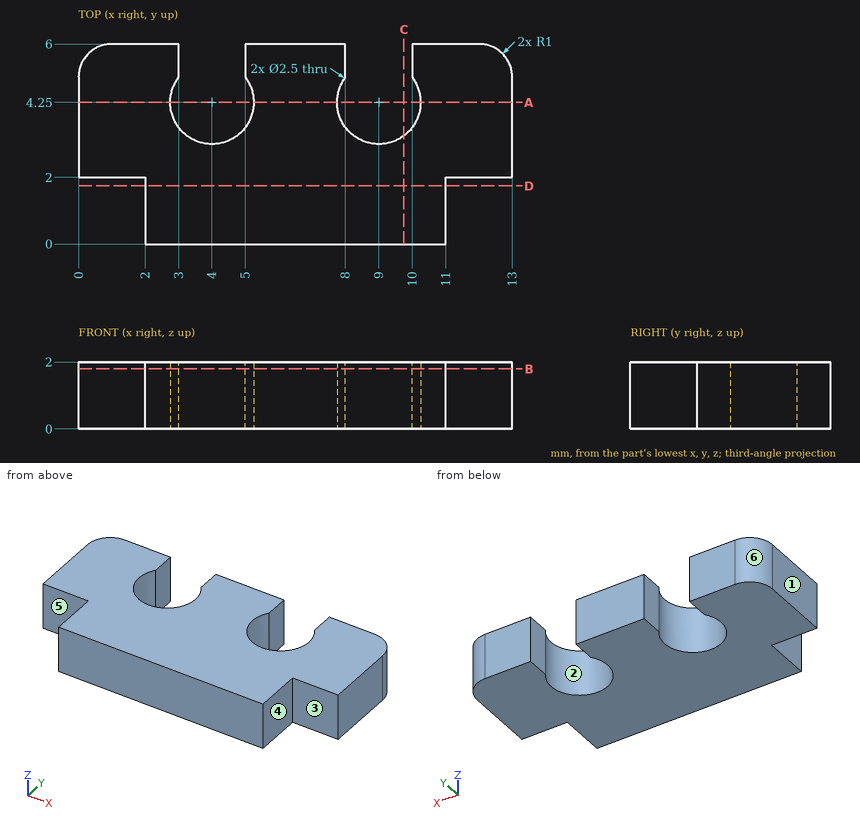
Geometry: see drawing. Coordinates: mm, zero at the bounding-box minimum. A direction names the side the tool comes from. Coordinates: 2 decimals unless noted, no trailing zeros. Order: outer loops, then holes, each group sorted by start corner. A loop starts at its lowest first (then second) coordinate and runs counter-clockwise, first axis right, second up. Notation, with made-up numbers: (38, 79.5) -> (57, 79.5) arc R28 cw to (57, 115.5) -> close; hole circle Ø9 at (89, 63). An arc over 180 degrees is marked (long way). Write each question's results on one line, items separated by ' | '. Start each with the question number.
1) Cut plane B-B, the plane z = 1.8. Output: boundary loops of the cut face in (x, y), and give its area (3 significant figures).
2) Cut plane C-C, the plane x = 9.75. Output: boundary loops of the cut face in (y, z), and give its area (3 significant figures).
3) Cut plane D-D, the plane y = 1.75. Output: boundary loops of the cut face in (x, z), and give its area (3 significant figures).
4) Set-up query: the marked faces 4, 5 and 6. Return all of +Z, -Z, +X, -X, +Y, -Y with unobstructed straight access to the full face (end or side cutting, diameter ignored); none if empty.
5) Mould query, pull axis X, two halves, no side actions, for the marked faces 1, 2 and 3. Classes: released by +X, released by -X, zero draft, split by the parting line, or undercut.
6) First-contact query: pin 1 (0.5 mm diameter, centred on y = 5.5, z = 1.5, fed in from -X); pin 2 (0.8 mm diameter, centred on y = 5.5, z = 1, fed in from +X) (3 decimals); pin 3 (2 mm diameter, centred on x = 4, y = 4.25, fed in from +Z). Flat tips, straight axial feed; report the tip coordinate or a pass-through.
7) Cut plane A-A, the plane y = 4.25. Output: boundary loops of the cut face in (x, z).
8) Material intervals for line 1 along X through (y, z) = (4.25, 1.25); line 2 along X through (y, z) = (5.3, 1.85); line 3 along Y through (x, z) = (4.25, 1.4), sorted ascending.
Checks:
1) outline: (0, 2) -> (2, 2) -> (2, 0) -> (11, 0) -> (11, 2) -> (13, 2) -> (13, 5) arc R1 ccw to (12, 6) -> (10, 6) -> (10, 5) arc R1.25 cw (long way) to (8, 5) -> (8, 6) -> (5, 6) -> (5, 5) arc R1.25 cw (long way) to (3, 5) -> (3, 6) -> (1, 6) arc R1 ccw to (0, 5) -> close | area: 57.2 mm^2
2) outline: (0, 0) -> (3.25, 0) -> (3.25, 2) -> (0, 2) -> close | area: 6.50 mm^2
3) outline: (2, 0) -> (11, 0) -> (11, 2) -> (2, 2) -> close | area: 18.0 mm^2
4) face 4: +Z, -Z, +X, -Y | face 5: +Z, -Z, -X, -Y | face 6: +Z, -Z, -X, +Y
5) face 1: released by -X | face 2: undercut | face 3: zero draft
6) pin 1: x = 0.03 | pin 2: x = 12.995 | pin 3: through
7) outline: (0, 0) -> (2.75, 0) -> (2.75, 2) -> (0, 2) -> close; (5.25, 0) -> (7.75, 0) -> (7.75, 2) -> (5.25, 2) -> close; (10.25, 0) -> (13, 0) -> (13, 2) -> (10.25, 2) -> close
8) line 1: 0 to 2.75, 5.25 to 7.75, 10.25 to 13 | line 2: 0.05 to 3, 5 to 8, 10 to 12.95 | line 3: 0 to 3.03
